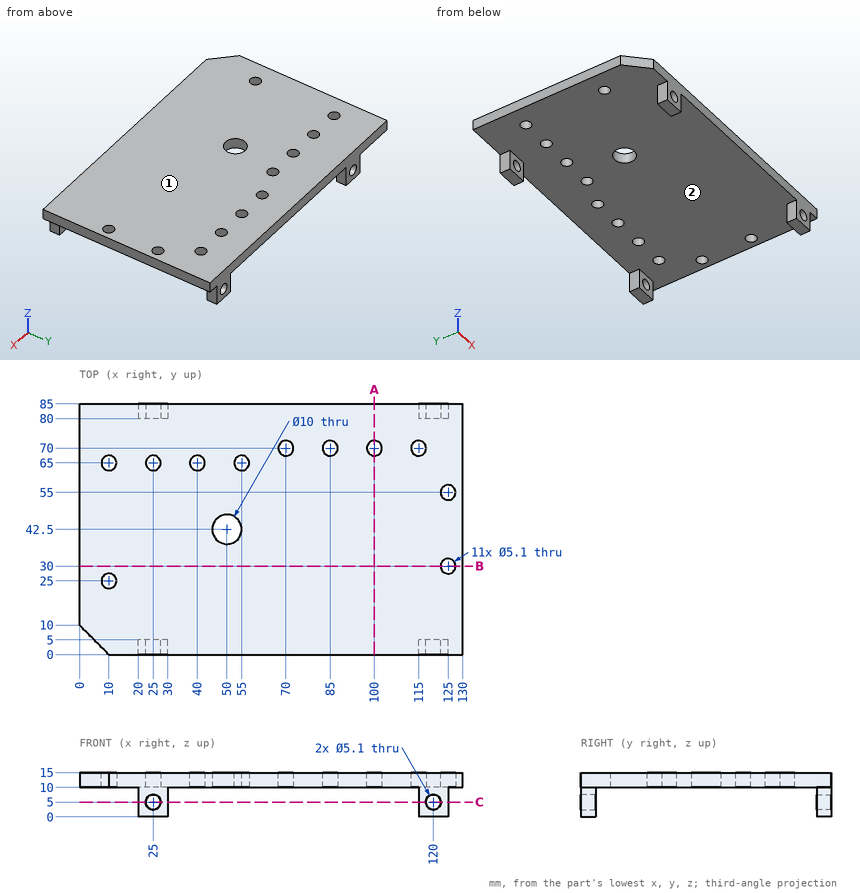
Print and shaded views of the part. All mm, measured from the part's lowest x, y and z. Round coordinates to 2 decimals unless told otherwise and drop trailing zeros. Write each loop counter-clockwise with the first axis right and the second up, starting at its lowest first coordinate (ties: lowest second). Pieces come first, ordered by that corner, then holes. Notation, with made-up numbers: (-28, -38.5) - (1, -38.5) arc R16 cw to (1, -24.5) - close; hole circle Ø11 at (-35, 65.25). An arc over 180 degrees is marked (long way). Use CSV: the item, a comma, the result in double quotes. Start each with the question number.
Item 1: Band-saw the part on C-C (z = 5). State how many separate pieces and enclosed holes the cut face has, and give its area (3 significant figures).
Item 2: Two-plate mould, pull along Y, no slides. Class the marked faces 1 and 2: released by +Y, released by -Y, zero draft, split by the parting line, or undercut.
Item 3: Band-saw the part on A-A (x = 100). Write the cut outline in (y, z).
Item 4: Pin check, flat tips, straight feed: P1, Ø4, axis at y = 81.5, z = 3, coming from the -X side; P2, Ø3, axis at x = 28.5, y = 51, coming from the -Z side; P3, Ø8, axis at x = 120, z = 5, coming from the +Y side; P4, Ø2.5, axis at y = 83, z = 7, coming from the +X side. Stop position of each tip, or through.
Item 5: Drill centre lines: L1, parallel to Y at x = 125, z = 11.5; L2, parallel to Y at x = 28, z = 2.75; L3, parallel to X at y = 65, z = 11.2. Where is each one in solid material? Low to high. Write a range as [from, to].
Item 6: Band-saw the part on B-B (y = 30). Write the cut outline in (x, z).
Checked values:
1,separate pieces,"8"
1,enclosed holes,"0"
1,area,"98.0 mm²"
2,face 1,"zero draft"
2,face 2,"undercut"
3,outline,"(0, 10) - (67.45, 10) - (67.45, 15) - (0, 15) - close; (72.55, 10) - (85, 10) - (85, 15) - (72.55, 15) - close"
4,P1,"stops at x = 20"
4,P2,"stops at z = 10"
4,P3,"stops at y = 85"
4,P4,"stops at x = 125"
5,L1,"y = [0, 27.45], [32.55, 52.45], [57.55, 85]"
5,L2,"y = [0, 5], [80, 85]"
5,L3,"x = [0, 7.45], [12.55, 22.45], [27.55, 37.45], [42.55, 52.45], [57.55, 130]"
6,outline,"(0, 10) - (122.45, 10) - (122.45, 15) - (0, 15) - close; (127.55, 10) - (130, 10) - (130, 15) - (127.55, 15) - close"
